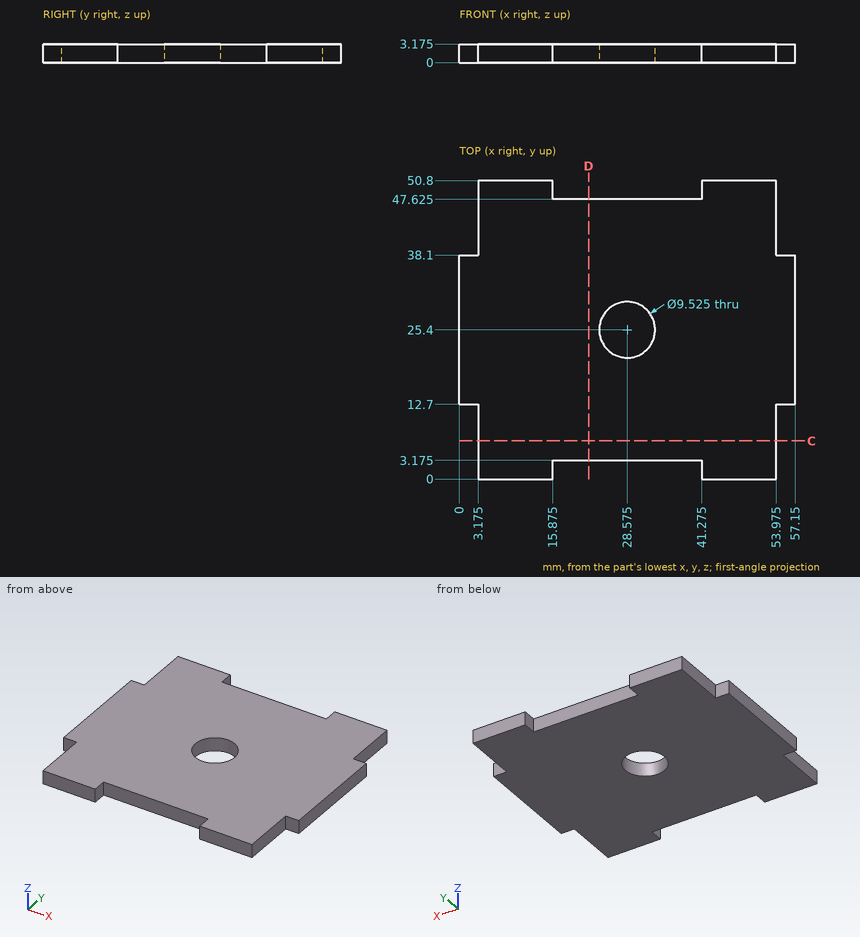
Verification items for this drawing (mm, ordinates from the low corner). Give positions to 0.01 mm unless a question says otherwise; leave off trailing zeros. Loops run counter-clockwise (first coordinate to the right, second up) from the corner with the lowest first, then second, coordinate; pieces in that order, holes last. Notation, with made-up numbers: M 44.5,80.5 L 63.5,80.5 A23 cw 63.5,101.5 Z; hole C 14.25,-25.5 d6. An arc over 180 degrees is marked long. Answer as a JSON object with one key per item and string values. Group by question number.
Q1. Cross-section at D-D on x = 22. Record the cut outline in (y, z) (3 decimals), then the cut area to 3 significant figures.
Q2. Cross-section at C-C on y = 6.5. Record the cut outline in (x, z) (3 decimals).
Q3. Go/stop test with flat-tipped pins: P1, Ø1, axis at y = 43, z = 2, coming from the -X side (3 decimals); P2, Ø1, axis at y = 7, z = 1.5, coming from the +X side (3 decimals); P3, Ø1.6, axis at x = 56, z = 2, coming from the -Y side. Record where each tip stops, or that it passes through.
Q4. Material ranges on line 1 along X through (y, z) = (25.5, 1.05); line 2 along X through (y, z) = (8.5, 0.95) (3 decimals); line 3 along X through (y, z) = (21, 1.35), recorded low to high. Write a range as [from, to].
Evaluation:
{
 "1": {"outline": "M 3.175,0 L 47.625,0 L 47.625,3.175 L 3.175,3.175 Z", "area": "141 mm2"},
 "2": {"outline": "M 3.175,0 L 53.975,0 L 53.975,3.175 L 3.175,3.175 Z"},
 "3": {"P1": "stops at x = 3.175", "P2": "stops at x = 53.975", "P3": "stops at y = 12.7"},
 "4": {"line 1": "x = [0, 23.81], [33.34, 57.15]", "line 2": "x = [3.175, 53.975]", "line 3": "x = [0, 26.75], [30.4, 57.15]"}
}
